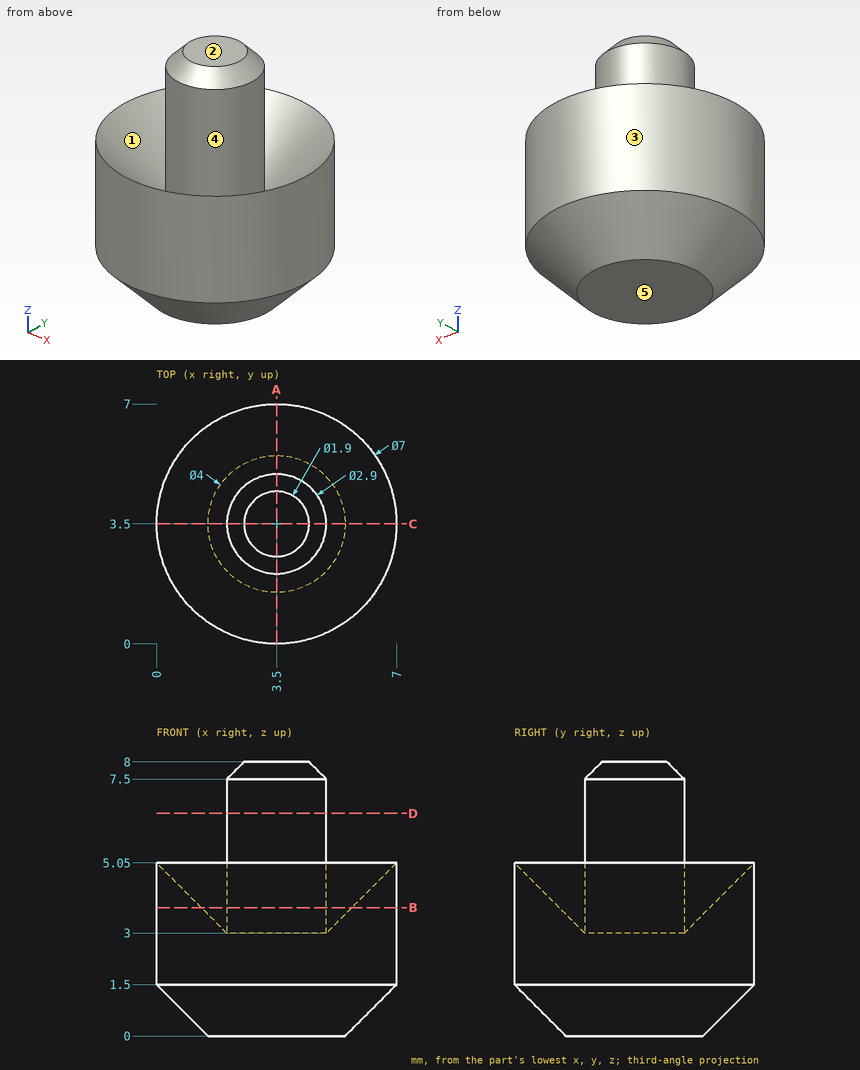
Geometry check sheet. Reference: drawing and pictorial views, mm from the part's lowest x, y, z. A direction names the side the tool comes from. Round coordinates to 2 decimals unless told otherwise and drop trailing zeros. Loops run counter-clockwise (first coordinate to the right, second up) from the corner with the lowest first, then second, coordinate; pieces in that order, holes last. Notation, with made-up numbers: (12.5, -14.5) -> (51.5, -14.5) arc R18 ccw to (51.5, 12.5) -> close; hole circle Ø2 at (-18, 82). An arc over 180 degrees is marked (long way). Answer as a JSON object with one key per item and string values. Group by question number.
Item 1: Set-up check for the marked faces 4 and 5: record each of +Z, -Z, +X, -X, +Y, -Y from which the full face is reachable in a straight line by a thin tool's end or side.
Item 2: Thickness scan on line 1 along X through (y, z) = (3, 3.5); line 2 along X through (y, z) = (4.5, 4.75); line 3 along Y through (x, z) = (4.5, 3.25). Record the ranges inside material, lowest first.
Item 3: Release check for a two-part mould opening along Y. For the marked faces 1, 2 and 3 record: pulls with the +Y half, pulls with the -Y half, needs draft (parallel to the pull), parting line crosses it, or undercut.
Item 4: Depth check by flat-ended pin: pin 1 Ø1 at (x, z) = (2.5, 3) entering from -Y; pin 2 Ø4 at (x, z) = (1, 6) entering from +Y; pin 3 Ø1.5 at (x, y) = (0.5, 6) entering from +Z. Enter the tip coordinate at first touch or a pass-through.
Item 5: Cross-section at D-D, the plane z = 6.5. Record the cut outline in (x, y), plus the area to 3 significant figures.
Item 6: Cross-section at A-A, the plane x = 3.5. Record the cut outline in (y, z), plus the area to 3 significant figures.
Item 7: Cross-section at B-B, the plane z = 3.75. Record the cut outline in (x, y).
Determined:
{
 "1": {"face 4": "+Z", "face 5": "-Z, +X, -X, +Y, -Y"},
 "2": {"line 1": "x = 0.04 to 1.62, 2.14 to 4.86, 5.38 to 6.96", "line 2": "x = 0.15 to 0.46, 2.45 to 4.55, 6.54 to 6.85", "line 3": "y = 0.15 to 2.13, 2.45 to 4.55, 4.87 to 6.85"},
 "3": {"face 1": "undercut", "face 2": "needs draft", "face 3": "parting line crosses it"},
 "4": {"pin 1": "stops at y = 0.04", "pin 2": "stops at y = 6.92", "pin 3": "stops at z = 5.05"},
 "5": {"outline": "circle Ø2.9 at (3.5, 3.5)", "area": "6.61 mm²"},
 "6": {"outline": "(0, 1.5) -> (1.5, 0) -> (5.5, 0) -> (7, 1.5) -> (7, 5.05) -> (4.95, 3) -> (4.95, 7.5) -> (4.45, 8) -> (2.55, 8) -> (2.05, 7.5) -> (2.05, 3) -> (0, 5.05) -> close", "area": "37.2 mm²"},
 "7": {"outline": "circle Ø7 at (3.5, 3.5); circle Ø2.9 at (3.5, 3.5); hole circle Ø4.4 at (3.5, 3.5)"}
}
